Part model, mm, in its own coordinate system. Face numbers are marked on the shaded views. Give positions to 0.01 mm unless a question says otherwise; leave off trailing zeros. Order: outer loops, then holes, each group sorted by start corner. A loop starts at its lowest first (then second) coordinate and runs counter-clockwise, first axis right, second up. Notation, with made-up numbers: M 34.5,78.25 L 43.5,78.25 A22 ccw 43.5,94.25 Z; hole C 10.5,10 d3. An arc over 180 degrees is marked long. Return JSON: item names as keys, results as strings.
from build123d import *

# Parameters (mm, degrees)
SKETCH1_W           = 100
SKETCH1_H           = 60
SKETCH1_R           = 2.3
BOSS_EXTRUDE1_DEPTH = 15
SKETCH2_R           = 9
CUT_EXTRUDE1_DEPTH  = 200


with BuildPart() as part:
    # Sketch1 → Boss-Extrude1 (new body)
    with BuildSketch(Plane.XY):
        Rectangle(SKETCH1_W, SKETCH1_H)
        with Locations((-40, -20)):
            Circle(SKETCH1_R, mode=Mode.SUBTRACT)
        with Locations(Location((40, -20, 0), (0, 0, 180))):
            Circle(SKETCH1_R, mode=Mode.SUBTRACT)
        with Locations((40, 20)):
            Circle(SKETCH1_R, mode=Mode.SUBTRACT)
        with Locations(Location((-40, 20, 0), (0, 0, 180))):
            Circle(SKETCH1_R, mode=Mode.SUBTRACT)
    extrude(amount=BOSS_EXTRUDE1_DEPTH)

    # Sketch2 → Cut-Extrude1 (cut, symmetric)
    with BuildSketch(Plane.ZY.offset(50)):
        Circle(SKETCH2_R)
    extrude(amount=CUT_EXTRUDE1_DEPTH, both=True, mode=Mode.SUBTRACT)


solid = part.part
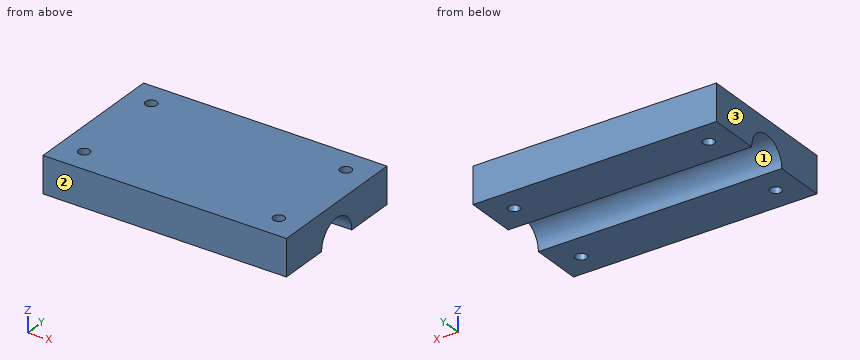
Q1. Two-plate mould, pull along Y, no slides. Class the marked faces 1, 2 and 3: +Y half, -Y half, draft (parallel to the pull), parting line (faces both ways), or undercut.
Established:
{"face 1": "undercut", "face 2": "-Y half", "face 3": "draft"}
Q2. Band-saw the part on B-B (z = 4.5). Give the cut face in (x, y).
Established:
{"outline": "M -50,-30 L 50,-30 L 50,-7.79 L -50,-7.79 Z; M -50,7.79 L 50,7.79 L 50,30 L -50,30 Z; hole C -40,-20 d4.6; hole C -40,20 d4.6; hole C 40,-20 d4.6; hole C 40,20 d4.6"}
Q3. Pin check, flat tips, straight feed: pin 1 (6 mm diameter, centred on x = 40, y = 20, fed in from +Z); pin 2 (3 mm diameter, centred on x = 39, y = -1.5, fed in from -Z). Stop position of each tip, or through.
Established:
{"pin 1": "stops at z = 15", "pin 2": "stops at z = 8.49"}
Q4. Band-saw the part on D-D (y = 0). Give the cut face in (x, z).
Established:
{"outline": "M -50,9 L 50,9 L 50,15 L -50,15 Z"}
Q5. Band-saw the part on A-A (x = -40). Give the cut face in (y, z).
Established:
{"outline": "M -30,0 L -22.3,0 L -22.3,15 L -30,15 Z; M -17.7,0 L -9,0 A9 cw 9,0 L 17.7,0 L 17.7,15 L -17.7,15 Z; M 22.3,0 L 30,0 L 30,15 L 22.3,15 Z"}
Q6. Band-saw the part on C-C (y = 20). Give the cut face in (x, z), then the cut area to 3 significant figures.
Established:
{"outline": "M -50,0 L -42.3,0 L -42.3,15 L -50,15 Z; M -37.7,0 L 37.7,0 L 37.7,15 L -37.7,15 Z; M 42.3,0 L 50,0 L 50,15 L 42.3,15 Z", "area": "1,360 mm²"}
Q7. Probe line 1 along Y through (x, z) = (22.5, 0.5); line 2 along Y through (x, z) = (40, 10.25); line 3 along Y through (x, z) = (-40, 5). List the from-to ranges inside material, lowest first.
Established:
{"line 1": "y = -30 to -8.99, 8.99 to 30", "line 2": "y = -30 to -22.3, -17.7 to 17.7, 22.3 to 30", "line 3": "y = -30 to -22.3, -17.7 to -7.48, 7.48 to 17.7, 22.3 to 30"}
